Solid Edge part; units mm, degrees
sketch "Sketch1" plane through (0, 0, 0) normal (0, -1, 0) x (1, 0, 0)
  arc A0 (0, 208.4456) -> (0, -97.0939) centre (0, 55.6758) ccw
  line L0 (0, 208.4456) -> (0, -97.0939)
revolve "RevolvedProtrusion1" add sketch "Sketch1" angle 360 about axis through (0, 0, 208.4456) along (0, 0, -1)
sketch "Sketch2" plane through (0, 0, 0) normal (0, -1, 0) x (1, 0, 0)
  line L0 (-68.8191, 42.5325) -> (-34.4095, 111.3516)
  line L1 (-34.4095, 111.3516) -> (42.5325, 111.3516)
extrude "Cutout1" cut sketch "Sketch2" along normal through all and the other way through all material side at (-51.659, 0, 76.9644)
sketch "Sketch3" plane through (0, 0, 0) normal (0, -1, 0) x (1, 0, 0)
  line L0 (68.8191, 68.8191) -> (34.4095, 0)
  line L1 (-42.5325, 0) -> (34.4095, 0)
extrude "Cutout2" cut sketch "Sketch3" along normal through all and the other way through all material side at (51.659, 0, 34.3872)
pattern_circular "Pattern1" count 5 over 360 about axis through (0, 0, 0) along (0, 0, 1) of "Cutout1", "Cutout2"
Model file for the job. Use its own axes, mm. Give positions to 0.01 mm unless a question says otherwise; leave off trailing zeros. Loops run counter-clockwise (first coordinate to the right, second up) from the corner with the lowest first, then second, coordinate; pieces in that order, holes last. Notation, with made-up numbers: (-13, 3.25) - (29, 3.25) arc R31 cw to (29, 41.25) - close; hole circle Ø9 at (81, -17). An arc over 180 degrees is marked (long way). One line per item, written item: value. Start each with the question number.
1. Pin check, flat tips, straight feed: pin 1 (2 mm diameter, centred on x = -23.5, z = 51, fed in from -Y); pin 2 (1.5 mm diameter, centred on x = -31.5, z = 36, fed in from -Y); pin 3 (4 mm diameter, centred on x = -43, z = 21.5, fed in from +Y). Stop position of each tip, or through.
2. Slice it at D-D (z = 76). List the corners of the cut face in (x, y), plus the area to 3 significant figures.
3. Slice it at B-B (z = 46). List the corners of the cut face in (x, y).
4. Slice it at A-A (y = -34). List the corners of the cut face in (x, z), plus the area to 3 significant figures.
5. Slice it at C-C (x = 8). List the corners of the cut face in (y, z), plus the area to 3 significant figures.
6. Probe L1, parallel to Y at x = 22, z = 23; L2, parallel to Z at x = 58, y = -5.5; L3, parallel to X at y = -30, z = 48.5. List the from-to ranges inside material, lowest first. Write a range as from..to.
Solution:
1. pin 1: stops at y = -60.89
1. pin 2: stops at y = -47.02
1. pin 3: stops at y = 20.88
2. outline: (-52.09, -37.84) - (19.89, -61.23) - (64.38, 0) - (19.89, 61.23) - (-52.09, 37.84) - close
2. area: 9,860 mm^2
3. outline: (-67.09, -5.34) - (-25.81, -62.15) - (-15.66, -65.45) - (51.14, -43.75) - (57.41, -35.11) - (57.41, 35.11) - (51.14, 43.75) - (-15.66, 65.45) - (-25.81, 62.15) - (-67.09, 5.34) - close
4. outline: (-57.77, 64.63) - (-17.83, 0) - (6.71, 0) - (46.8, 24.77) - (57.77, 46.72) - (17.83, 111.35) - (-6.71, 111.35) - (-46.8, 86.58) - close
4. area: 8,510 mm^2
5. outline: (-65.45, 60.62) - (-33.58, 0) - (33.58, 0) - (65.45, 60.62) - (38.78, 111.35) - (-38.78, 111.35) - close
5. area: 11,300 mm^2
6. L1: y = -41.12..41.12
6. L2: z = 47.18..79.86
6. L3: x = -50.71..58.66
